from build123d import *

# Parameters (mm, degrees)
F1_DEPTH = 1.5
F2_R     = 2
F3_R     = 2.4
F4_DEPTH = 25


with BuildPart() as f1:
    # F0 (on Front) → F1 (new body, symmetric)
    with BuildSketch(Plane.XZ):
        with BuildLine():
            ThreePointArc((0, -50), (-16.484532, -47.204451), (-31.125732, -39.130408))
            Line((-31.125732, -39.130408), (-35, -44.00103))
            Line((-35, -44.00103), (-35, -65))
            Line((-35, -65), (35, -65))
            Line((35, -65), (35, -44.00103))
            Line((35, -44.00103), (31.125732, -39.130408))
            ThreePointArc((31.125732, -39.130408), (16.484532, -47.204451), (0, -50))
        make_face()
    extrude(amount=F1_DEPTH, both=True)

    # F2
    f2_edges = [f1.edges().sort_by_distance(p)[0] for p in [
        (31.125732, 0, -39.130408),
        (35, 0, -44.00103),
        (35, 0, -65),
        (-31.125732, 0, -39.130408),
        (-35, 0, -44.00103),
        (-35, 0, -65),
    ]]
    fillet(f2_edges, radius=F2_R)

    # F3 (on face) → F4 (cut)
    with BuildSketch(Plane.XZ.offset(1.5)):
        with Locations((-25, -55)):
            Circle(F3_R)
        with Locations((25, -55)):
            Circle(F3_R)
    extrude(amount=-F4_DEPTH, mode=Mode.SUBTRACT)


solid = f1.part
Model file for the job. Use its own axes, mm. Give positions to 0.01 mm unless a question says otherwise; leave off trailing zeros. Write each loop counter-clockwise with the first axis right and the second up, starting at its lowest first coordinate (ties: lowest second). Pieces come first, ordered by that corner, then holes. Notation, with made-up numbers: (12.25, -26) - (30.25, -26) arc R7 ccw to (30.25, -14) - close; hole circle Ø4 at (52, 71). An arc over 180 degrees is marked (long way). Answer as CSV lines item,"result".
1. Band-saw the part on C-C (x = 14). Write the cut outline in (y, z), and give its area (3 significant figures).
Responses:
outline,"(-1.5, -65) - (1.5, -65) - (1.5, -48) - (-1.5, -48) - close"
area,"51.0 mm2"
2. Two-plate mould, pull along X, no slides. Class faces 1 (the face through (26.11, -0.02, -57.13)), 2 (the face through (-35, 0, -54)), 3 (the face through (34.885, 0.021, -44.031)): +X half, -X half, draft (parallel to the pull), parting line (faces both ways), or undercut.
Responses:
face 1,"undercut"
face 2,"-X half"
face 3,"+X half"
3. Band-saw the part on A-A (y = 1). Write the cut outline in (x, z), and give its area (3 significant figures).
Responses:
outline,"(-35, -63) arc R2 ccw to (-33, -65) - (33, -65) arc R2 ccw to (35, -63) - (35, -44.7) arc R2 ccw to (34.57, -43.45) - (32.35, -40.67) arc R2 ccw to (29.6, -40.3) arc R50 cw to (0, -50) arc R50 cw to (-29.6, -40.3) arc R2 ccw to (-32.35, -40.67) - (-34.57, -43.45) arc R2 ccw to (-35, -44.7) - close; hole circle Ø4.8 at (-25, -55); hole circle Ø4.8 at (25, -55)"
area,"1,290 mm2"
4. Band-saw the part on D-D (x = -10.5). Write the cut outline in (y, z).
Responses:
outline,"(-1.5, -65) - (1.5, -65) - (1.5, -48.89) - (-1.5, -48.89) - close"
5. Drill centre lines: L1, parallel to X at y = 0.75, z = -54.5; L2, parallel to X at y = 0.55, z = -56.75; L3, parallel to Z at x = 25, y = 0.25. Where is each one in solid material? Low to high. Write a range as [from, to].
Responses:
L1,"x = [-35, -27.35], [-22.65, 22.65], [27.35, 35]"
L2,"x = [-35, -26.64], [-23.36, 23.36], [26.64, 35]"
L3,"z = [-65, -57.4], [-52.6, -43.3]"
6. Band-saw the part on B-B (x = 25). Write the cut outline in (y, z), and give its area (3 significant figures).
Responses:
outline,"(-1.5, -65) - (1.5, -65) - (1.5, -57.4) - (-1.5, -57.4) - close; (-1.5, -52.6) - (1.5, -52.6) - (1.5, -43.3) - (-1.5, -43.3) - close"
area,"50.7 mm2"
